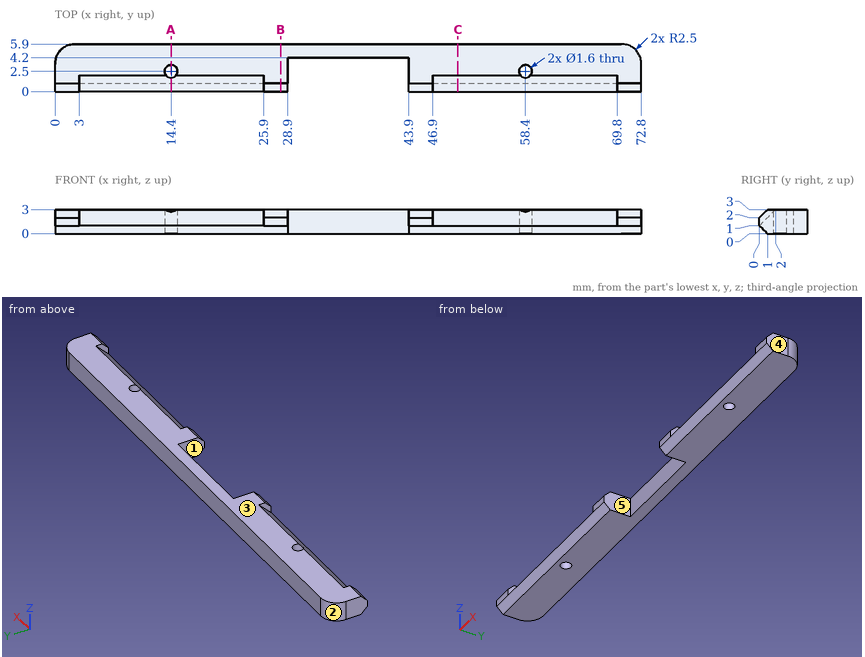
Part print with two shaded views. Sizes in mm from the minimum x, y, z corner. A direction names the side the tool comes from. Coordinates: 2 decimals unless noted, no trailing zeros. Write each loop counter-clockwise with the first axis right and the second up, starting at its lowest first coordinate (ties: lowest second). Pieces come first, ordered by that corner, then holes.
(1) Cut at B-B on x = 28. List the corners of the cut face in (y, z).
(2) Cut at A-A on x = 14.4. List the corners of the cut face in (y, z), and give its area (3 significant figures).
(3) Mould opens along X. For the marked faces 3, 4 and 5 say: pulls with the +X half, pulls with the -X half, needs draft (parallel to the pull), parting line crosses it, or undercut.
(4) 3-axis set-ups, long thin cutter, end or side, ignore diameter. For the marked faces 1 and 2: which of +Z, -Z, +X, -X, +Y, -Y reach the whole face in a straight line?
(5) Pin check, flat tips, straight feed: pin 1 Ø2.5 at (x, y) = (14.4, 2.5) entering from +Z; pin 2 Ø1.5 at (x, z) = (52, 2.5) entering from -Y; pin 3 Ø0.9 at (x, z) = (34, 2) entering from -Y. Stop position of each tip, or through.
(6) Drill centre lines: line 1 (X direction, y = 2.5, z = 0.75); line 2 (X direction, y = 1.2, z = 1.3); line 3 (Y direction, x = 32.5, z = 1.95). Where is each one in solid material? Low to high.
(7) Cut at C-C on x = 50. List the corners of the cut face in (y, z).
Working result:
1. outline: (0, 1) - (1, 0) - (5.9, 0) - (5.9, 3) - (1, 3) - (0, 2) - close
2. outline: (0, 1) - (1, 0) - (1.7, 0) - (1.7, 2.7) - close; (3.3, 0) - (5.9, 0) - (5.9, 3) - (3.3, 3) - close
2. area: 10.4 mm2
3. face 3: needs draft
3. face 4: pulls with the +X half
3. face 5: undercut
4. face 1: +Z, -Z, -Y
4. face 2: +Z, -Z, -X, +Y
5. pin 1: stops at z = 3
5. pin 2: stops at y = 0.75
5. pin 3: stops at y = 4.2
6. line 1: x = 0 to 13.6, 15.2 to 28.9, 43.9 to 57.6, 59.2 to 72.8
6. line 2: x = 0 to 28.9, 43.9 to 72.8
6. line 3: y = 4.2 to 5.9
7. outline: (0, 1) - (1, 0) - (5.9, 0) - (5.9, 3) - (2, 3) - close
